Autodesk Inventor part; units mm, degrees
ref_plane "YZ Plane" through (0, 0, 0) normal (1, 0, 0) x (0, 1, 0)
ref_plane "XZ Plane" through (0, 0, 0) normal (0, 1, 0) x (-1, 0, 0)
ref_plane "XY Plane" through (0, 0, 0) normal (0, 0, 1) x (1, 0, 0)
sketch "Sketch1" plane through (0, 0, 0) normal (1, 0, 0) x (0, 1, 0)
  line L0 (-45, 135) -> (45, 135)
  line L1 (45, 135) -> (45, -135)
  line L2 (45, -135) -> (-45, -135)
  line L3 (-45, -135) -> (-45, 135)
  line L4 (-45, 135) -> (45, -135) construction
  line L5 (45, 135) -> (-45, -135) construction
  point P0 (0, 0)
  dimension "d0" = 90
  dimension "d1" = 270
extrude "Extrusion1" add sketch "Sketch1" along normal blind 10
sketch "Sketch2" plane through (0, 0, 0) normal (-1, 0, 0) x (0, 0, 1)
  line L0 (-135, -45) -> (-135, 45)
  line L1 (135, -45) -> (-135, -45)
  line L2 (135, 45) -> (135, -45)
  line L3 (-135, 45) -> (135, 45)
  line L4 (0, 45) -> (0, -5)
  line L5 (145, 25) -> (-145, 25)
  line L6 (-145, 25) -> (-145, -35)
  line L7 (-145, -35) -> (145, -35)
  line L8 (145, -35) -> (145, 25)
  line L9 (145, 25) -> (-145, -35) construction
  line L10 (-145, 25) -> (145, -35) construction
  point P0 (-135, -35)
  point P1 (-135, 25)
  point P2 (135, 25)
  point P3 (135, -35)
  dimension "d8" = 90
  dimension "d9" = 50
  dimension "d10" = 60
  dimension "d11" = 290
  dimension "d12" = 270
extrude "Extrusion2" add sketch "Sketch2" against normal blind 10 contours L7 L6 L5 L0 | L2 L5 L8 L7
properties part number "03_Tam_top_vs_bottom" material "Stainless Steel, Austenitic"
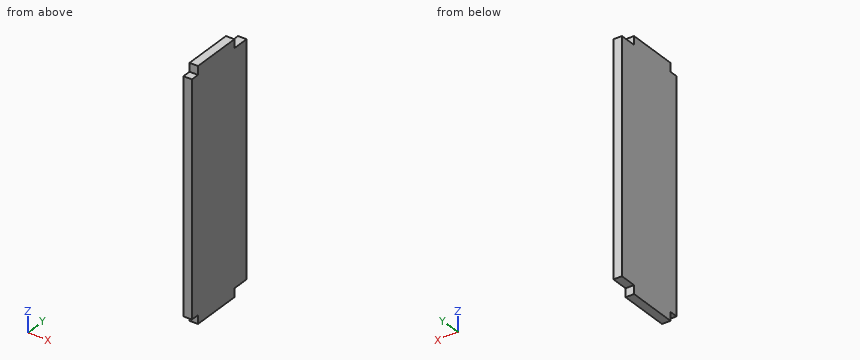
Input: part model. Units: mm. Frame: model coordinates. Coordinates: 2 decimals unless noted, no trailing zeros. Loops run counter-clockwise (first coordinate to the right, second up) from the corner with the lowest first, then second, coordinate; pieces in that order, holes last. Notation, with made-up numbers: (-23.5, 42.5) -> (30.5, 42.5) arc R10 cw to (30.5, 47.5) -> close; hole circle Ø2 at (80.5, 50.5). An arc over 180 degrees is marked (long way). Write each question's results on one line, items separated by ' | '. Start each with the question number.
Q1. Ray query, line 1 (Z direction, x = 9, y = 35). Return the intervals inside material, ascending. Write a range as from..to.
Q2. Pin query (flat end, axial travel): pin 1 (5 mm diameter, centred on x = 5.5, y = 31.5, fed in from +Z); pin 2 (5 mm diameter, centred on x = 7.5, y = 33, fed in from -Z); pin 3 (3 mm diameter, centred on x = 4, z = 138.5, fed in from -Y). Return the tip coordinate at first contact, or that it passes through.
Q3. Section A-A, the plane x = 2. Return the cut outline in (y, z).
Q4. Section B-B, the plane y = 31.5. Return the cut outline in (x, z), plus the area to 3 significant figures.
Found:
1) line 1: -135..135
2) pin 1: z = 135 | pin 2: z = -135 | pin 3: y = -35
3) outline: (-45, -135) -> (-35, -135) -> (-35, -145) -> (25, -145) -> (25, -135) -> (45, -135) -> (45, 135) -> (25, 135) -> (25, 145) -> (-35, 145) -> (-35, 135) -> (-45, 135) -> close
4) outline: (0, -135) -> (10, -135) -> (10, 135) -> (0, 135) -> close | area: 2,700 mm2
